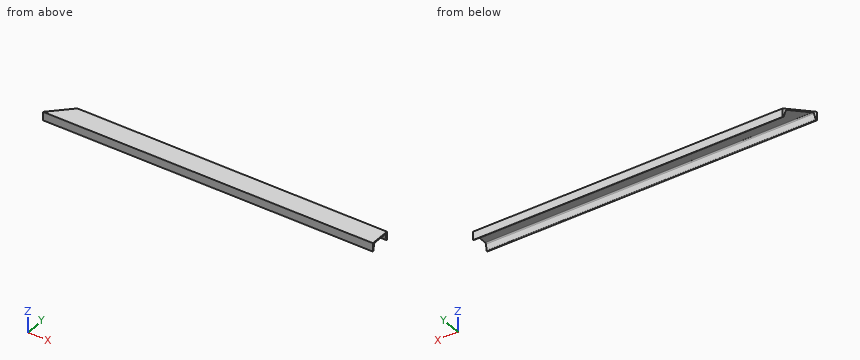
```python
from build123d import *

# Parameters (mm, degrees)
F1_DEPTH = 2489.2
F3_DEPTH = 63.4248


with BuildPart() as f1:
    # F0 (on Right) → F1 (new body)
    with BuildSketch(Plane.YZ):
        with BuildLine():
            Line((76.2, 0), (-76.2, 0))
            Line((-76.2, 0), (-76.2, -63.4238))
            ThreePointArc((-76.2, -63.4238), (-72.574321, -62.102069), (-70.649887, -58.757061))
            Line((-70.649887, -58.757061), (-63.124886, -15.566335))
            ThreePointArc((-63.124886, -15.566335), (-59.952782, -10.052651), (-53.976459, -7.874))
            Line((-53.976459, -7.874), (53.976459, -7.874))
            ThreePointArc((53.976459, -7.874), (59.952782, -10.052651), (63.124886, -15.566335))
            Line((63.124886, -15.566335), (70.649887, -58.757061))
            ThreePointArc((70.649887, -58.757061), (72.574321, -62.102069), (76.2, -63.4238))
            Line((76.2, -63.4238), (76.2, 0))
        make_face()
    extrude(amount=F1_DEPTH)

    # F2 (on face) → F3 (cut, through all)
    with BuildSketch(Plane.XY):
        Polygon((0, 76.2), (0, -76.2), (152.4, 76.2), align=None)
    extrude(amount=-F3_DEPTH, mode=Mode.SUBTRACT)


solid = f1.part
```
The listing builds one solid part. Answer for the finished solid, in the listing's coordinates (mm). Round coordinates to 2 decimals unless told otherwise and drop trailing zeros. Loops run counter-clockwise (first coordinate to the right, second up) from the corner with the lowest first, then second, coordinate; pieces in that order, holes last. Notation, with made-up numbers: (89, 34) - (117, 34) arc R8 cw to (117, 41) - close; hole circle Ø3 at (50, -1.5). An arc over 180 degrees is marked (long way). Use one line per item in the form item = value. Start each with the question number.
1. The part is cut by section B-B on z = -25.5. Determine the outline of the cut face in (x, y), then the cut area to 3 significant figures.
2. The part is cut by section A-A on x = 2319.5. Determine the outline of the cut face in (y, z), then the cut area to 3 significant figures.
3. The part is cut by section C-C on y = 14.5. Determine the outline of the cut face in (x, z), then the cut area to 3 significant figures.
4. Consider line 1 (Y direction, x = 1987, z = -17); line 2 (Z direction, x = 2273, y = -35.5); line 3 (Y direction, x = 232, z = -51.5). Determine where each line is inside the solid, lowest interval first. Write a range as [from, to].
5. Given pin 1 Ø1 at (x, y) = (874.5, 37.5) entering from -Z, flat-ended and moving along its own axis, determine where the tip first touches the part or whether it passes through.
Geometry check:
q1.outline = (0, -76.2) - (2489.2, -76.2) - (2489.2, -64.86) - (11.34, -64.86) - close; (141.06, 64.86) - (2489.2, 64.86) - (2489.2, 76.2) - (152.4, 76.2) - close
q1.area = 54,700 mm^2
q2.outline = (-76.2, -63.42) arc R5.63 ccw to (-70.65, -58.76) - (-63.12, -15.57) arc R9.29 cw to (-53.98, -7.87) - (53.98, -7.87) arc R9.29 cw to (63.12, -15.57) - (70.65, -58.76) arc R5.63 ccw to (76.2, -63.42) - (76.2, 0) - (-76.2, 0) - close
q2.area = 2,280 mm^2
q3.outline = (90.7, -7.87) - (2489.2, -7.87) - (2489.2, 0) - (90.7, 0) - close
q3.area = 18,900 mm^2
q4.line_1 = [-76.2, -63.37], [63.37, 76.2]
q4.line_2 = [-7.87, 0]
q4.line_3 = [-76.2, -69.39], [69.39, 76.2]
q5.pin_1 = -7.87
